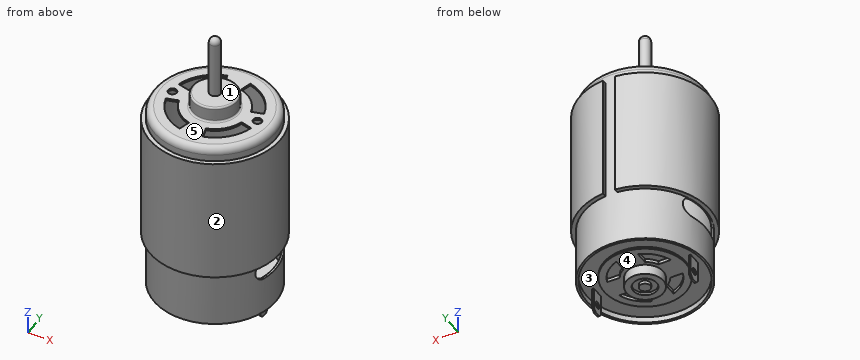
Autodesk Inventor part; units mm, degrees
ref_plane "Work Plane1" through (0, 0, -26.875) normal (0, 0, -1) x (-1, 0, 0)
ref_plane "Work Plane2" through (18, 0, 0) normal (1, 0, 0) x (0, 1, 0)
ref_plane "Work Plane3" through (0, 0, 24.625) normal (0, 0, 1) x (1, 0, 0)
sketch "Sketch1" plane through (0, 0, 0) normal (0, 0, 1) x (1, 0, 0)
  circle A0 centre (0, 0) radius 17.75
  dimension "d0" = 35.5
extrude "Extrusion1" add sketch "Sketch1" along normal mid plane 57.25
fillet "Fillet1" radius 2 1 edges at (-17.75, 0, 28.625)
shell "Shell1" thickness 0.62 removed faces 1 at (3.0438, 4.2648, -28.625)
sketch "Sketch2" plane through (0, 0, 28.625) normal (0, 0, 1) x (1, 0, 0)
  circle A0 centre (0, 0) radius 15.75
  circle A1 centre (0, 0) radius 6.5
  dimension "d5" = 13
extrude "Extrusion2" add sketch "Sketch2" along normal blind 4.5 contours A1
fillet "Fillet2" radius 0.5 2 edges at (-6.5, 0, 28.625) (-6.5, 0, 33.125)
sketch "Sketch3" plane through (0, 0, 33.125) normal (0, 0, 1) x (1, 0, 0)
  circle A0 centre (0, 0) radius 6
  circle A1 centre (0, 0) radius 1.6
  dimension "d9" = 3.2
extrude "Extrusion3" add sketch "Sketch3" along normal blind 18 contours A1
fillet "Fillet3" radius 1.6 1 edges at (-1.6, 0, 51.125)
sketch "Sketch4" plane through (0, 0, 28.625) normal (0, 0, 1) x (1, 0, 0)
  circle A0 centre (0, 0) radius 15.75
  point P0 (12.5, 0)
  dimension "d13" = 12.5
hole "Hole1" at (12.5, 0, 28.625) direction (0, 0, -1) diameter 2.5 depth 8 tip angle 118
mirror "Mirror1" about plane through (0, 0, 0) normal (1, 0, 0) of "Hole1"
sketch "Sketch5" plane through (0, 0, 28.625) normal (0, 0, 1) x (1, 0, 0)
  circle A0 centre (12.5, 0) radius 1.25
  circle A1 centre (0, 0) radius 7
  arc A2 (12.557, 3.3646) -> (3.3646, 12.557) centre (0, 0) ccw
  arc A3 (9.1763, 2.4588) -> (2.4588, 9.1763) centre (0, 0) ccw
  line L0 (0, 0) -> (3.3646, 12.557) construction
  line L1 (0, 0) -> (12.557, 3.3646) construction
  line L2 (2.4588, 9.1763) -> (3.3646, 12.557)
  line L3 (9.1763, 2.4588) -> (12.557, 3.3646)
  line L4 (0, 0) -> (12.5, 0) construction
  line L5 (0.151, 0.5634) -> (0.151, 14.7153) construction
  dimension "d21" = 15
  dimension "d22" = 15
  dimension "d23" = 13
  dimension "d24" = 9.5
extrude "Extrusion4" cut sketch "Sketch5" against normal blind 10 contours L3 A3 L2 A2
pattern_circular "Circular Pattern1" count 4 over 360 about axis through (0, 0, 0) along (0, 0, 1) of "Extrusion4"
ref_plane "Work Plane1" through (0, 0, -26.875) normal (0, 0, -1) x (-1, 0, 0)
sketch "Sketch6" plane through (0, 0, -26.875) normal (0, 0, -1) x (-1, 0, 0)
  circle A0 centre (0, 0) radius 17.13
extrude "Extrusion5" add sketch "Sketch6" against normal blind 0.62
sketch "Sketch7" plane through (0, 0, -26.875) normal (0, 0, -1) x (-1, 0, 0)
  circle A0 centre (0, 0) radius 17.13
  circle A1 centre (0, 0) radius 12
  dimension "d33" = 24
extrude "Extrusion6" add sketch "Sketch7" along normal blind 0.62 contours A1
sketch "Sketch8" plane through (0, 0, -27.495) normal (0, 0, -1) x (-1, 0, 0)
  circle A0 centre (0, 0) radius 12
  circle A1 centre (0, 0) radius 5.375
  dimension "d36" = 10.75
extrude "Extrusion7" add sketch "Sketch8" along normal blind 3 contours A1
sketch "Sketch9" plane through (0, 0, -30.495) normal (0, 0, -1) x (-1, 0, 0)
  circle A0 centre (0, 0) radius 5.375
  circle A1 centre (0, 0) radius 3.45
  dimension "d39" = 6.9
extrude "Extrusion8" cut sketch "Sketch9" against normal blind 0.8 contours A1
sketch "Sketch10" plane through (0, 0, -29.695) normal (0, 0, -1) x (-1, 0, 0)
  circle A0 centre (0, 0) radius 3.45
  circle A1 centre (0, 0) radius 1.6
  dimension "d42" = 3.2
extrude "Extrusion9" add sketch "Sketch10" along normal blind 1 contours A1
sketch "Sketch11" plane through (0, 0, -27.495) normal (0, 0, -1) x (-1, 0, 0)
  circle A0 centre (0, 0) radius 5.375
  circle A1 centre (0, 0) radius 12
  arc A2 (9.3591, 3.15) -> (3.15, 9.3591) centre (0, 0) ccw
  arc A3 (5.6857, 3.15) -> (3.15, 5.6857) centre (0, 0) ccw
  line L0 (3.15, 9.3591) -> (3.15, 5.6857)
  line L1 (5.6857, 3.15) -> (9.3591, 3.15)
  dimension "d45" = 3.15
  dimension "d46" = 3.15
  dimension "d47" = 9.875
  dimension "d48" = 6.5
extrude "Extrusion10" cut sketch "Sketch11" against normal blind 1 contours L1 A3 L0 A2
pattern_circular "Circular Pattern2" count 4 over 360 about axis through (0, 0, 0) along (0, 0, 1) of "Extrusion10"
sketch "Sketch12" plane through (0, 0, -26.875) normal (0, 0, -1) x (-1, 0, 0)
  circle A0 centre (0, 0) radius 12
  circle A1 centre (0, 0) radius 17.13
  line L0 (-14.5, 1.9) -> (-14, 1.9)
  line L1 (-14, 1.9) -> (-14, -1.9)
  line L2 (-14, -1.9) -> (-14.5, -1.9)
  line L3 (-14.5, -1.9) -> (-14.5, 1.9)
  line L4 (0, 0) -> (-16.9017, 0) construction
  point P0 (-14, 0)
  dimension "d54" = 0.5
  dimension "d55" = 3.8
  dimension "d56" = 14
extrude "Extrusion11" add sketch "Sketch12" along normal blind 7.2 contours L0 L1 L2 L3
chamfer "Chamfer1" distance 1 angle 45 2 edges at (14.25, 1.9, -34.075) (14.25, -1.9, -34.075)
sketch "Sketch13" plane through (14.5, -1.9, -26.875) normal (1, 0, 0) x (0, 0, -1)
  line L0 (7.2, 1) -> (7.2, 2.8)
  line L1 (4.2, 1.9) -> (6.2, 3.8) construction
  line L2 (4.2, 1.9) -> (6.2, 0) construction
  dimension "d61" = 3
hole "Hole2" at (14.5, 0, -31.075) direction (-1, 0, 0) diameter 2 depth 1 tip angle 118
mirror "Mirror2" about plane through (0, 0, 0) normal (1, 0, 0) of "Extrusion11", "Chamfer1", "Hole2"
ref_plane "Work Plane2" through (18, 0, 0) normal (1, 0, 0) x (0, 1, 0)
sketch "Sketch14" plane through (18, 0, 0) normal (1, 0, 0) x (0, 1, 0)
  arc A0 (-4.5554, -11.975) -> (-4.5554, -17.875) centre (-4.5554, -14.925) ccw
  arc A1 (5.2946, -17.875) -> (5.2946, -11.975) centre (5.2946, -14.925) ccw
  line L0 (-4.5554, -11.975) -> (5.2946, -11.975)
  line L1 (-4.5554, -17.875) -> (5.2946, -17.875)
  line L2 (17.75, -28.625) -> (-17.75, -28.625)
  line L3 (0, -28.625) -> (0, 20.5314) construction
  dimension "d70" = 10.75
  dimension "d71" = 5.9
  dimension "d72" = 9.85
extrude "Extrusion12" cut sketch "Sketch14" against normal through all
ref_plane "Work Plane3" through (0, 0, 24.625) normal (0, 0, 1) x (1, 0, 0)
sketch "Sketch15" plane through (0, 0, 24.625) normal (0, 0, 1) x (1, 0, 0)
  circle A0 centre (0, 0) radius 17.75
  arc A1 (-1.75, 18.9192) -> (1.75, 18.9192) centre (0, 0) ccw
  line L0 (-1.75, 18.9192) -> (-1.75, 17.6635)
  line L1 (1.75, 18.9192) -> (1.75, 17.6635)
  line L2 (0, 0) -> (0, 21.9354) construction
  dimension "d76" = 38
  dimension "d77" = 3.5
extrude "Extrusion13" add sketch "Sketch15" against normal blind 37 contours A0 L1 A1 L0
properties part number "FisherPriceMotor 550 motor" material "Steel, Mild"
Check sheet for the modelled part. Datum: model origin and axes. Units: mm. Face numbers are marked on the shaded views. A direction names the side the tool comes from. Round coordinates to 2 decimals unless told otherwise and drop trailing zeros. Loops run counter-clockwise (first coordinate to the right, second up) from the corner with the lowest first, then second, coordinate; pieces in that order, holes last. Notation, with made-up numbers: (61.5, -11) -> (84.5, -11) arc R24 cw to (84.5, 24) -> close; hole circle Ø3 at (66.25, 39). An arc over 180 degrees is marked (long way). Write item = value, one per line. Start each with the question number.
1) Release check for a two-part mould opening along X. For the marked faces 1, 2 and 3 record: released by +X, released by -X, zero draft, split by the parting line, or undercut.
2) Sectioned sample at D-D, the plane z = 42. Record the cut outline in (x, y), plus the area to 3 significant figures.
3) Set-up check for the marked faces 4 and 5: record each of +Z, -Z, +X, -X, +Y, -Y from which the full face is reachable in a straight line by a thin tool's end or side.
4) Sectioned sample at A-A, the plane z = -13.5. Record the cut outline in (x, y), plus the area to 3 significant figures.
5) Sectioned sample at C-C, the plane z = -23. Record the cut outline in (x, y), plus the area to 3 significant figures.
6) Gauge pin test, flat ends, axial feed: pin 1 Ø0.8 at (x, z) = (7, -27) entering from -Y; pin 2 Ø0.8 at (y, z) = (-8, -27) entering from -X; pin 3 Ø3 at (x, y) = (-6.5, 5.5) entering from -Z (3 decimals); pin 4 Ø12 at (y, z) = (-1.5, -14) entering from -X. Record the tip position at first contact, or that the pin passes through.
7) Thickness scan on probe 1 along Z at (x, y) = (-14.1, 0) (3 decimals); probe 2 along Y at (x, z) = (0, -27.55) (3 decimals); probe 3 along Y at (x, z) = (-0.5, 11). Record the ranges inside material, lowest first.
8) Sectioned sample at B-B, the plane y = 0. State how many separate pieces and enclosed holes the cut face has, plus the area to 3 significant figures.
Results are:
q1.face_1 = zero draft
q1.face_2 = split by the parting line
q1.face_3 = undercut
q2.outline = circle Ø3.2 at (0, 0)
q2.area = 8.04 mm^2
q3.face_4 = -Z
q3.face_5 = +Z
q4.outline = (-16.25, -7.14) arc R17.75 ccw to (16.25, -7.14) -> (15.57, -7.14) arc R17.13 cw to (-15.57, -7.14) -> close; (-15.91, 7.88) -> (-15.21, 7.88) arc R17.13 cw to (15.21, 7.88) -> (15.91, 7.88) arc R17.75 ccw to start
q4.area = 48.7 mm^2
q5.outline = circle Ø35.5 at (0, 0); hole circle Ø34.26 at (0, 0)
q5.area = 67.9 mm^2
q6.pin_1 = -16.48
q6.pin_2 = -16.04
q6.pin_3 = -27.495
q6.pin_4 = -19
q7.probe_1 = -34.075 to -32.075, -30.075 to -26.255, 28.005 to 28.625
q7.probe_2 = -17.75 to -17.13, -5.375 to 5.375, 17.13 to 17.75
q7.probe_3 = -18.99 to -17.12, 17.12 to 17.74
q8.separate_pieces = 6
q8.enclosed_holes = 0
q8.area = 360 mm^2
